```python
from build123d import *

# Parameters (mm, degrees)
SKETCH_1_R      = 2.5
EXTRUDE_1_DEPTH = 2


with BuildPart() as part:
    # Эскиз1 → Бобышка-Вытянуть1 (new body)
    with BuildSketch(Plane.XY):
        with BuildLine():
            Line((-14.033668667, -6.927741673), (9.836212535, -6.927741673))
            Line((9.836212535, -6.927741673), (9.836212535, 6.468384532))
            ThreePointArc((9.836212535, 6.468384532), (-1.939735679, 47.334627745), (-33.656179922, 75.668175974))
            ThreePointArc((-33.656179922, 75.668175974), (-42.372566631, 73.171176021), (-40.898194288, 64.224856542))
            ThreePointArc((-40.898194288, 64.224856542), (-23.309833652, 43.806018062), (-14.033668667, 18.503208773))
            Line((-14.033668667, 18.503208773), (-14.033668667, -6.927741673))
        make_face()
        Circle(SKETCH_1_R, mode=Mode.SUBTRACT)
    extrude(amount=EXTRUDE_1_DEPTH)


solid = part.part
```
Build history of the part. All positions in model axes, mm. A direction names the side the tool comes from. Round coordinates to 2 decimals unless told otherwise and drop trailing zeros. Write each loop counter-clockwise with the first axis right and the second up, starting at its lowest first coordinate (ties: lowest second). Pieces come first, ordered by that corner, then holes. Notation, with made-up numbers: (61, 16) -> (114, 16) arc R12 cw to (114, 30) -> close; hole circle Ø9 at (71, -7.75). An arc over 180 degrees is marked (long way). Put each result on its own line as item: value.
Item 1: Slice it at C-C, the plane x = 0. Give the cut face in (y, z), plus the area to 3 significant figures.
Here are the results:
outline: (-6.93, 0) -> (-2.5, 0) -> (-2.5, 2) -> (-6.93, 2) -> close; (2.5, 0) -> (44.07, 0) -> (44.07, 2) -> (2.5, 2) -> close
area: 92.0 mm^2
Item 2: Flat gauge pins, fed straight in: P1, Ø4, axis at x = -33, y = 58, coming from the -Z side; P2, Ø4.5, axis at x = 0, y = 0, coming from the -Z side. Where does each tip first touch, or does it go through?
Here are the results:
P1: stops at z = 0
P2: passes through
Item 3: Slice it at B-B, the plane y = 0. Give the cut face in (x, z).
Here are the results:
outline: (-14.03, 0) -> (-2.5, 0) -> (-2.5, 2) -> (-14.03, 2) -> close; (2.5, 0) -> (9.84, 0) -> (9.84, 2) -> (2.5, 2) -> close
Item 4: Slice it at A-A, the plane z = 0.6. Give the cut face in (x, y), plus the area to 3 significant figures.
Here are the results:
outline: (-40.9, 64.22) arc R75.33 cw to (-14.03, 18.5) -> (-14.03, -6.93) -> (9.84, -6.93) -> (9.84, 6.47) arc R76.8 ccw to (-33.66, 75.67) arc R6.82 ccw to start; hole circle Ø5 at (0, 0)
area: 1,870 mm^2
Item 5: Slice it at D-D, the plane x = -37. Give the cut face in (y, z), plus the area to 3 significant figures.
Here are the results:
outline: (60.85, 0) -> (76.33, 0) -> (76.33, 2) -> (60.85, 2) -> close
area: 31.0 mm^2
Item 6: Two-plate mould, pull along X, no slides. Class faces 3 (the face through (-0.54, -2.44, 0.99)), 4 (the face through (-42.297, 73.288, 0.986)), 5 (the face through (-11, 35, 2)), 6 (the face through (-23.5, 44.13, 0.99)): pulls with the +X half, pulls with the -X half, needs draft (parallel to the pull), parting line crosses it, or undercut.
Here are the results:
face 3: undercut
face 4: parting line crosses it
face 5: needs draft
face 6: pulls with the -X half
Item 7: Tool access for faces 1 (the face through (-14.034, 6, 1)), 2 (the face through (-1.62, 46.82, 0.99)): list every direction of +Z, -Z, +X, -X, +Y, -Y with a clear straight run to the whole face (end or side of a thin tool).
Here are the results:
face 1: +Z, -Z, -X, -Y
face 2: +Z, -Z, +X, +Y
Item 8: Wall check: probe 1 along X at (y, z) = (-1, 1.4); probe 2 along Y at (x, z) = (0, 1.5); probe 3 along X at (y, z) = (52, 0.5). Give the ranges that are in metal, low to high. Write a range as from..to.
Here are the results:
probe 1: x = -14.03..-2.29, 2.29..9.84
probe 2: y = -6.93..-2.5, 2.5..44.07
probe 3: x = -28.88..-5.12
